Here's how the part is built. I have some questions about the finished solid (model axes, mm). A direction names the side the tool comes from. Give positions to 0.01 mm unless a question says otherwise; leave off trailing zeros. Order: outer loops, then holes, each group sorted by start corner. A loop starts at its lowest first (then second) coordinate and runs counter-clockwise, first axis right, second up. Notation, with made-up numbers: M 50,-19 L 70,-19 A18 ccw 70,-7 Z; hole C 56,43 d5. An arc over 180 degrees is marked long. Use CSV: the item, a comma, the result in double quotes. Start each with the question number.
```python
from build123d import *

# Parameters (mm, degrees)
F0_W      = 2
F0_H      = 10
F1_DEPTH  = 0.3
F2_W      = 2
F2_H      = 2.65
F2_H_2    = 10
F3_DEPTH  = 0.2
F4_W      = 0.5
F4_H      = 7.5
F4_H_2    = 5.8
F4_W_2    = 2
F5_DEPTH  = 0.7
F6_W      = 3
F6_H      = 1.7
F6_H_2    = 1.6
F7_DEPTH  = 0.1
F8_W      = 0.475
F8_H      = 1.7
F8_H_2    = 1.6
F9_DEPTH  = 0.5
F10_W     = 0.5
F10_H     = 0.2
F10_W_2   = 2
F11_DEPTH = 0.3
F12_SCALE = 3


with BuildPart() as f1:
    # F0 (on Top) → F1 (new body)
    with BuildSketch(Plane.XY):
        Rectangle(F0_W, F0_H)
    extrude(amount=F1_DEPTH)

    # F2 (on face) → F3 (join)
    with BuildSketch(Plane.XY.offset(0.3)):
        with Locations((0, 6.325)):
            Rectangle(F2_W, F2_H)
        Rectangle(F2_W, F2_H_2)
        with Locations((0, -6.325)):
            Rectangle(F2_W, F2_H)
    extrude(amount=F3_DEPTH)

    # F4 (on face) → F5 (join)
    with BuildSketch(Plane.XY.offset(0.5)):
        with Locations((-1.25, 3.9)):
            Rectangle(F4_W, F4_H)
        with Locations((1.25, 3.9)):
            Rectangle(F4_W, F4_H)
        with Locations((-1.25, -4.75)):
            Rectangle(F4_W, F4_H_2)
        with Locations((1.25, -4.75)):
            Rectangle(F4_W, F4_H_2)
        with Locations((0, 3.9)):
            Rectangle(F4_W_2, F4_H)
        with Locations((0, -4.75)):
            Rectangle(F4_W_2, F4_H_2)
    extrude(amount=F5_DEPTH)

    # F6 (on face) → F7 (join)
    with BuildSketch(Plane.XY.offset(1.2)):
        with Locations((0, 6.8)):
            Rectangle(F6_W, F6_H)
        with Locations((0, -6.85)):
            Rectangle(F6_W, F6_H_2)
    extrude(amount=F7_DEPTH)

    # F8 (on face) → F9 (join)
    with BuildSketch(Plane.XY.offset(1.3)):
        with Locations((-1.2625, 6.8)):
            Rectangle(F8_W, F8_H)
        with Locations((1.2625, 6.8)):
            Rectangle(F8_W, F8_H)
        with Locations((-1.2625, -6.85)):
            Rectangle(F8_W, F8_H_2)
        with Locations((1.2625, -6.85)):
            Rectangle(F8_W, F8_H_2)
    extrude(amount=F9_DEPTH)

    # F10 (on face) → F11 (cut)
    with BuildSketch(Plane(origin=(0, 0, 0.3), x_dir=(1, 0, 0), z_dir=(0, 0, -1))):
        with Locations((1.25, 7.25)):
            Rectangle(F10_W, F10_H)
        with Locations((-1.25, 7.25)):
            Rectangle(F10_W, F10_H)
        with Locations((0, 7.25)):
            Rectangle(F10_W_2, F10_H)
    extrude(amount=-F11_DEPTH, mode=Mode.SUBTRACT)


with BuildPart() as f1_1:
    # F12: moved
    add(f1.part.scale(F12_SCALE))


solid = f1_1.part
```
Q1. For P1, Ø2, axis at x = -0.5, y = 5, coming from the +Z side; P2, Ø0.7, axis at y = -22.5, z = 1, coming from the -X side; P3, Ø0.5, axis at x = -1, y = -22.5, coming from the -Z side, each with a flat end and sliding along its axis, tell me the tip position at first contact or that it passes through.
Q2. We'd pull the mould along X, two halves only. Please class faces 6 (the face through (0, -22.5, 0.9)), 7 (the face through (3.075, 20, 5)), 8 (the face through (-4.5, -16, 3)), 9 (the face through (0, -21, 3.9)): pulls with the +X half, pulls with the -X half, needs draft (parallel to the pull), parting line crosses it, or undercut.
Q3. For faces 1 (the face through (3.075, -21, 5)), 2 (the face through (0, 19, 0.9)), 3 (the face through (-3.8, -22.5, 1.5)), 4 (the face through (0, -22.95, 3)), 5 (the face through (0, -5.55, 3)), which set-ups out of +Z, -Z, +X, -X, +Y, -Y let a thin tool reach every point of the face, with its end or its side?
Q4. Imagine slicing it at D-D, the plane y = 20. Please give me the cut outline in (x, z) (3 decimals), then the cut area to 3 significant figures.
Q5. Imagine slicing it at A-A, the plane z = 4.8. Please give me the cut outline in (x, y) (3 decimals).
Q6. Imagine slicing it at C-C, the plane z = 3.05. Please give me the cut outline in (x, y).
Q7. Imagine slicing it at B-B, the plane x = 3.5. Please give me the cut outline in (y, z).
Q8. I need wall thicknesses on line 1 (Y direction, x = 0.25, z = 3.5); line 2 (Y direction, x = 2, z = 1.25); line 3 (Z direction, x = -4, y = 3.5). Which ranges of each line are inside material? Lowest first, please. Write a range as [from, to].
Reply:
1,P1,"stops at z = 3.6"
1,P2,"stops at x = -3"
1,P3,"stops at z = 0.9"
2,face 6,"needs draft"
2,face 7,"undercut"
2,face 8,"pulls with the -X half"
2,face 9,"undercut"
3,face 1,"+Z, +Y, -Y"
3,face 2,"-Z, +X, -X, +Y"
3,face 3,"-Z, -X, +Y, -Y"
3,face 4,"+Z, -Z, +X, -X, -Y"
3,face 5,"+Z, +X, -X"
4,outline,"M -4.5,1.5 L -3,1.5 L -3,0.9 L 3,0.9 L 3,1.5 L 4.5,1.5 L 4.5,5.4 L 3.075,5.4 L 3.075,3.9 L -3.075,3.9 L -3.075,5.4 L -4.5,5.4 Z"
4,area,"29.5 mm^2"
5,outline,"M -4.5,-22.95 L -3.075,-22.95 L -3.075,-18.15 L -4.5,-18.15 Z; M -4.5,17.85 L -3.075,17.85 L -3.075,22.95 L -4.5,22.95 Z; M 3.075,-22.95 L 4.5,-22.95 L 4.5,-18.15 L 3.075,-18.15 Z; M 3.075,17.85 L 4.5,17.85 L 4.5,22.95 L 3.075,22.95 Z"
6,outline,"M -4.5,-22.95 L 4.5,-22.95 L 4.5,-5.55 L -4.5,-5.55 Z; M -4.5,0.45 L 4.5,0.45 L 4.5,22.95 L -4.5,22.95 Z"
7,outline,"M -22.95,1.5 L -22.05,1.5 L -22.05,1.8 L -21.45,1.8 L -21.45,1.5 L -5.55,1.5 L -5.55,3.6 L -18.15,3.6 L -18.15,5.4 L -22.95,5.4 Z; M 0.45,1.5 L 22.95,1.5 L 22.95,5.4 L 17.85,5.4 L 17.85,3.6 L 0.45,3.6 Z"
8,line 1,"y = [-22.95, -5.55], [0.45, 22.95]"
8,line 2,"y = [-22.95, -22.05], [-21.45, 22.95]"
8,line 3,"z = [1.5, 3.6]"
